Design review of the part built by this model. Coordinates are the model's own, in mm. Give positions to 0.01 mm unless a question says otherwise; leave off trailing zeros. Order: outer loops, then holes, each group sorted by start corner. A loop starts at its lowest first (then second) coordinate and runs counter-clockwise, first axis right, second up. Notation, with made-up numbers: (-10.5, -27) -> (37.5, -27) arc R12 cw to (37.5, -13) -> close; hole circle Ø11 at (-15, 84.25). An arc over 180 degrees is marked (long way). Return JSON: item names as keys, results as strings.
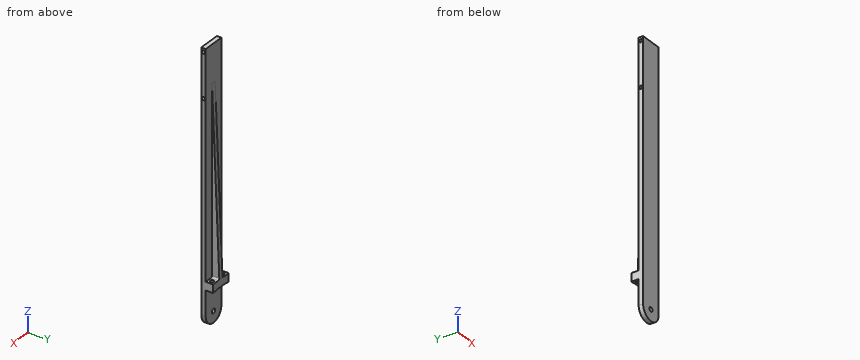
```python
from build123d import *

# Parameters (mm, degrees)
ESQUISSE1_W             = 30
ESQUISSE1_H             = 6
BOSS_EXTRU_1_DEPTH      = 300
BOSS_EXTRU_2_DEPTH      = 3
BOSS_EXTRU_2_DEPTH_BACK = 3
ESQUISSE4_W             = 30
ESQUISSE4_H             = 16
BOSS_EXTRU_3_DEPTH      = 10
ESQUISSE7_R             = 3
BOSS_EXTRU_5_DEPTH      = 6
ESQUISSE8_R             = 2.1
ENL_V_MAT_EXTRU_1_DEPTH = 12
ENL_V_START             = -18
ESQUISSE8_2_R           = 2.1
ENL_V_MAT_EXTRU_3_DEPTH = 12
BOSS_EXTRU_6_DEPTH      = 16
ESQUISSE10_R            = 2.5
ENL_V_MAT_EXTRU_4_DEPTH = 302.920519342
CONG_1_R                = 2


with BuildPart() as part:
    # Esquisse1 → Boss.-Extru.1 (new body)
    with BuildSketch(Plane.XY):
        with Locations((15, 3)):
            Rectangle(ESQUISSE1_W, ESQUISSE1_H)
    extrude(amount=BOSS_EXTRU_1_DEPTH)

    # Esquisse3 → Boss.-Extru.2 (add, two sides: drawn at the far end of the back side and taken through both)
    with BuildSketch(Plane(origin=(15, 0, 0), x_dir=(0, 0, -1), z_dir=(1, 0, 0)).offset(-BOSS_EXTRU_2_DEPTH_BACK)):
        Polygon((-250, 6), (0, 16), (0, 6), align=None)
    extrude(amount=BOSS_EXTRU_2_DEPTH + BOSS_EXTRU_2_DEPTH_BACK)

    # Esquisse4 → Boss.-Extru.3 (add)
    with BuildSketch(Plane(origin=(0, 0, 0), x_dir=(-1, 0, 0), z_dir=(0, 0, -1))):
        with Locations((-15, 8)):
            Rectangle(ESQUISSE4_W, ESQUISSE4_H)
    extrude(amount=BOSS_EXTRU_3_DEPTH)

    # Esquisse7 → Boss.-Extru.5 (add)
    with BuildSketch(Plane.XZ):
        with BuildLine():
            Line((0, -10), (0, -45))
            ThreePointArc((0, -45), (15, -60), (30, -45))
            Line((30, -45), (30, -10))
            Line((30, -10), (0, -10))
        make_face()
        with Locations(Location((15, -45, 0), (0, 0, 270))):
            Circle(ESQUISSE7_R, mode=Mode.SUBTRACT)
    extrude(amount=-BOSS_EXTRU_5_DEPTH)

    # Esquisse8 → Enlèv. mat.-Extru.1 (cut)
    with BuildSketch(Plane.ZY):
        with Locations((295, 3)):
            Circle(ESQUISSE8_R)
        with Locations((235, 3)):
            Circle(ESQUISSE8_R)
    extrude(amount=-ENL_V_MAT_EXTRU_1_DEPTH, mode=Mode.SUBTRACT)

    # Esquisse8<2> → Enlèv. mat.-Extru.3 (cut)
    with BuildSketch(Plane.ZY.offset(ENL_V_START)):
        with Locations((295, 3)):
            Circle(ESQUISSE8_2_R)
        with Locations((235, 3)):
            Circle(ESQUISSE8_2_R)
    extrude(amount=-ENL_V_MAT_EXTRU_3_DEPTH, mode=Mode.SUBTRACT)

    # Esquisse9 → Boss.-Extru.6 (add)
    with BuildSketch(Plane(origin=(0, 16, 0), x_dir=(1, 0, 0), z_dir=(0, 1, 0))):
        with BuildLine():
            Line((0, 11.131400334), (0, 0))
            Line((0, 0), (30, 0))
            Line((30, 0), (30, 11.131400334))
            ThreePointArc((30, 11.131400334), (15, 10), (0, 11.131400334))
        make_face()
    extrude(amount=-BOSS_EXTRU_6_DEPTH)

    # Esquisse10 → Enlèv. mat.-Extru.4 (cut, through all)
    with BuildSketch(Plane.XY):
        with Locations((5, 11)):
            Circle(ESQUISSE10_R)
        with Locations((25, 11)):
            Circle(ESQUISSE10_R)
    extrude(amount=-ENL_V_MAT_EXTRU_4_DEPTH, mode=Mode.SUBTRACT)

    # Congé1
    # the kernel refuses this fillet: 2 mm, written as the material it adds along each edge
    with BuildSketch(Plane(origin=(12, 16, 0), x_dir=(-1, 0, 0), z_dir=(0, -1, 0))) as cong_1_piece_1_section:
        with BuildLine():
            CenterArc((CONG_1_R, -CONG_1_R), CONG_1_R, 90, 90)
            Line((0, -CONG_1_R), (0, 0))
            Line((0, 0), (CONG_1_R, 0))
        make_face()
    cong_1_piece_1 = extrude(amount=15, mode=Mode.PRIVATE)
    cong_1_piece_1 = split(cong_1_piece_1, bisect_by=Plane(origin=(11.546773045, 15.973945238, 0.651369053), z_dir=(0, -0.9992009587217895, -0.03996803834887158)), keep=Keep.TOP, mode=Mode.PRIVATE)
    add(cong_1_piece_1)
    with BuildSketch(Plane(origin=(18, 16, 0), x_dir=(1, 0, 0), z_dir=(0, -1, 0))) as cong_1_piece_2_section:
        with BuildLine():
            CenterArc((CONG_1_R, CONG_1_R), CONG_1_R, 180, 90)
            Line((0, CONG_1_R), (0, 0))
            Line((0, 0), (CONG_1_R, 0))
        make_face()
    cong_1_piece_2 = extrude(amount=15, mode=Mode.PRIVATE)
    cong_1_piece_2 = split(cong_1_piece_2, bisect_by=Plane(origin=(18.453226955, 15.973945238, 0.651369053), z_dir=(0, -0.9992009587217895, -0.03996803834887158)), keep=Keep.TOP, mode=Mode.PRIVATE)
    add(cong_1_piece_2)


solid = part.part
```
Item 1: Add section A-A (x = 15). Give the boundary of the cut face in (y, z), plus the area to 3 significant figures.
Result set:
{"outline": "(0, -60) -> (6, -60) -> (6, -48) -> (0, -48) -> close; (0, -42) -> (6, -42) -> (6, -10) -> (16, -10) -> (16, 0) -> (6, 250) -> (6, 300) -> (0, 300) -> close", "area": "3,470 mm^2"}
Item 2: Add section C-C (z = 131.5). Give the boundary of the cut face in (x, y).
Result set:
{"outline": "(0, 0) -> (30, 0) -> (30, 6) -> (18, 6) -> (18, 10.74) -> (12, 10.74) -> (12, 6) -> (0, 6) -> close"}
Item 3: Add section B-B (z = 227.5). Give the boundary of the cut face in (x, y).
Result set:
{"outline": "(0, 0) -> (30, 0) -> (30, 6) -> (18, 6) -> (18, 6.9) -> (12, 6.9) -> (12, 6) -> (0, 6) -> close"}
Item 4: Wall thickness on L1, parallel to X at y = 11, z = -7.25; L2, parallel to Y at x = 9, z = 235; L3, parallel to X at y = 2.8, z = -45: over which ranges is each line inside the solid? List them lowest first. Write a range as [from, to].
Result set:
{"L1": "x = [0, 2.5], [7.5, 22.5], [27.5, 30]", "L2": "y = [0, 0.9], [5.1, 6]", "L3": "x = [0, 12], [18, 30]"}
Item 5: For pin 1 (5 mm diameter, centred on y = 12.5, z = 84.5, fed in from +X); pin 2 (5 mm diameter, centred on y = 10.5, z = 76, fed in from -X); pin 3 (8 mm diameter, centred on x = 15, z = -45, fed in from +Y), all flat-tipped, find the tip position at first contact; note any pin that passes through.
Result set:
{"pin 1": "stops at x = 18", "pin 2": "stops at x = 12", "pin 3": "stops at y = 6"}
